For this review, take the finished solid that the model builds, in its own axes (mm). Give positions to 0.01 mm unless a question says otherwise; leave off trailing zeros. Order: outer loops, then holes, each group sorted by start corner. A loop starts at its lowest first (then second) coordinate and runs counter-clockwise, first axis right, second up.
from build123d import *

# Parameters (mm, degrees)
ESBO_O1_W                 = 400
ESBO_O1_H                 = 360
RESSALTO_EXTRUS_O1_DEPTH  = 2.5
FILETE1_R                 = 10
ESBO_O2_R                 = 2.65
CORTE_EXTRUS_O1_DEPTH     = 270.118932816
ESPELHAR2_COPY_1_SKETCH_R = 2.65
ESPELHAR2_COPY_1_DEPTH    = 270.118932816
ESBO_O3_W                 = 5
ESBO_O3_H                 = 20
CORTE_EXTRUS_O2_DEPTH     = 270.118932816
PADR_O_LINEAR1_COUNT      = 3
PADR_O_LINEAR1_PITCH      = 40
CORTE_EXTRUS_O3_DEPTH     = 270.118932816


with BuildPart() as part:
    # Esbo_o1 → Ressalto-extrus_o1 (new, symmetric)
    with BuildSketch(Plane(origin=(0, 0, 0), x_dir=(0, 0, -1), z_dir=(1, 0, 0))):
        Rectangle(ESBO_O1_W, ESBO_O1_H)
    extrude(amount=RESSALTO_EXTRUS_O1_DEPTH, both=True)

    # Filete1
    filete1_edges = [part.edges().sort_by_distance(p)[0] for p in [
        (0, -180, -200),
        (0, -180, 200),
        (0, 180, 200),
        (0, 180, -200),
    ]]
    fillet(filete1_edges, radius=FILETE1_R)

    # Esbo_o2 → Corte-extrus_o1 (cut, through all)
    with BuildSketch(Plane(origin=(2.5, 0, 0), x_dir=(0, 0, -1), z_dir=(1, 0, 0))):
        with Locations((-190, -170)):
            Circle(ESBO_O2_R)
        with Locations((-170, -170)):
            Circle(ESBO_O2_R)
        with Locations((-150, -170)):
            Circle(ESBO_O2_R)
        with Locations((-190, -150)):
            Circle(ESBO_O2_R)
        with Locations((-190, -130)):
            Circle(ESBO_O2_R)
    corte_extrus_o1 = extrude(amount=-CORTE_EXTRUS_O1_DEPTH, mode=Mode.SUBTRACT)

    # Espelhar1: Corte-extrus_o1 across plane
    add(corte_extrus_o1.mirror(Plane.XY), mode=Mode.SUBTRACT)

    # Espelhar2: Corte-extrus_o1 across plane
    add(corte_extrus_o1.mirror(Plane.ZX), mode=Mode.SUBTRACT)

    # Espelhar2 copy 1 sketch → Espelhar2 copy 1 (cut, through all)
    with BuildSketch(Plane(origin=(2.5, 0, 0), x_dir=(0, 0, 1), z_dir=(1, 0, 0))):
        with Locations((-190, -170)):
            Circle(ESPELHAR2_COPY_1_SKETCH_R)
        with Locations((-170, -170)):
            Circle(ESPELHAR2_COPY_1_SKETCH_R)
        with Locations((-150, -170)):
            Circle(ESPELHAR2_COPY_1_SKETCH_R)
        with Locations((-190, -150)):
            Circle(ESPELHAR2_COPY_1_SKETCH_R)
        with Locations((-190, -130)):
            Circle(ESPELHAR2_COPY_1_SKETCH_R)
    extrude(amount=-ESPELHAR2_COPY_1_DEPTH, mode=Mode.SUBTRACT)

    # Esbo_o3 → Corte-extrus_o2 (cut, through all)
    with BuildSketch(Plane(origin=(2.5, 0, 0), x_dir=(0, 0, -1), z_dir=(1, 0, 0))):
        with Locations((-137.5, -63)):
            Rectangle(ESBO_O3_W, ESBO_O3_H)
    corte_extrus_o2 = extrude(amount=-CORTE_EXTRUS_O2_DEPTH, mode=Mode.SUBTRACT)

    # Padr_o linear1: Corte-extrus_o2 ×3
    with Locations(*[(0, i * PADR_O_LINEAR1_PITCH, 0) for i in range(1, PADR_O_LINEAR1_COUNT)]):
        add(corte_extrus_o2, mode=Mode.SUBTRACT)

    # Esbo_o4 → Corte-extrus_o3 (cut, through all)
    with BuildSketch(Plane.ZY.offset(2.5)):
        with BuildLine():
            Line((30, -150), (-30, -150))
            ThreePointArc((-30, -150), (-50, -130), (-30, -110))
            Line((-30, -110), (30, -110))
            ThreePointArc((30, -110), (50, -130), (30, -150))
        make_face()
    extrude(amount=-CORTE_EXTRUS_O3_DEPTH, mode=Mode.SUBTRACT)


solid = part.part
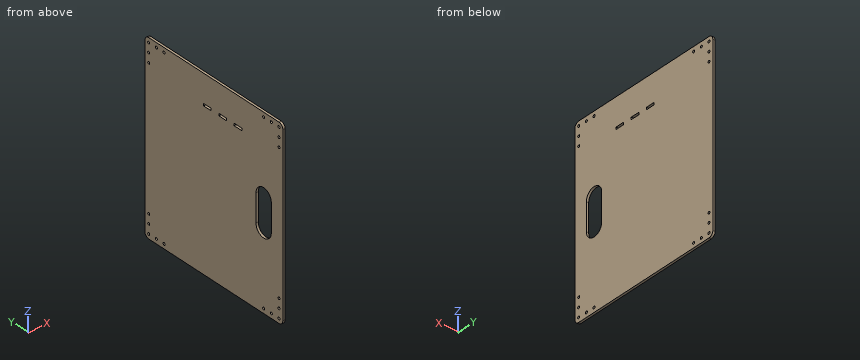
1) We need section A-A on z = -22.5. Give the boundary of the cut face in (x, y).
Answer sheet:
outline: (-2.5, -180) - (2.5, -180) - (2.5, -150) - (-2.5, -150) - close; (-2.5, -110) - (2.5, -110) - (2.5, 180) - (-2.5, 180) - close
2) Clearance check with a flat-ended pin moving along its axis: pin 1 (3 mm diameter, centred on y = -170, z = 150, fed in from -X). State where the tip first meets the part, or that it passes through.
Answer sheet:
pin 1: passes through
3) We need section B-B on x = 1.2. Count the separate pieces of the cut face and the enclosed holes in it, then the cut area to 3 significant figures.
Answer sheet:
separate pieces: 1
enclosed holes: 24
area: 140,000 mm2
4) To check wall thickness, follow line 1 (Z direction, x = -1.45, y = 130); line 2 (Y direction, x = 0.2, z = -170); line 3 (Z direction, x = 2.25, y = 16). State the ranges of each line that lie inside material, in increasing order.
Answer sheet:
line 1: z = -200 to -192.65, -187.35 to 187.35, 192.65 to 200
line 2: y = -180 to -172.65, -167.35 to 167.35, 172.65 to 180
line 3: z = -200 to 135, 140 to 200
